For this review, take the finished solid that the model builds, in its own axes (mm). A direction names the side the tool comes from. Give positions to 0.01 mm unless a question says otherwise; leave off trailing zeros. Loops run counter-clockwise (first coordinate to the right, second up) from the corner with the lowest first, then second, coordinate; pieces in that order, holes last. Notation, with made-up numbers: (-16.75, 0) -> (28.25, 0) arc R21 ccw to (28.25, 12) -> close; hole circle Ø11 at (54.25, 30). An arc over 180 degrees is marked (long way). Answer as CSV lines item,"result". Start each with the question number.
Item 1: For L1, parallel to X at y = 35, z = 42.5; L2, parallel to Y at x = 90, z = 13; L3, parallel to Z at x = 5, y = 9, list the stretches that pass through material, from the lowest coordinate up. Write a range as from..to.
Item 2: Add section C-C on y = 32. State the section outline as (x, z) points.
Item 3: Clearance check with flat-ended pins moving along their axes: P1, Ø12, axis at x = 75, z = 18.5, coming from the +Y side; P2, Ø2, axis at y = 50.5, z = 39.5, coming from the +X side; P3, Ø3, axis at x = 16, z = 32.5, coming from the +Y side. State where each tip first meets the part, or that it passes through.
Item 4: Machinability: for faces 5 (the face through (94, 32, 41)), 6 (the face through (60, 55, 25)), 7 (the face through (35, 35, 38)), 8 (the face through (82, 3, 25)), which of the approach directions +Z, -Z, +X, -X, +Y, -Y give a long, thin tool a straight path to every point of the face, cutting with its end or side? Answer none if there is none.
Item 5: The part is to be moulded in two halves that separate along Y. For faces 1 (the face through (56.51, 4.19, 24.65)), 2 (the face through (86.4, 32.3, 20.2)), 3 (the face through (80, 41, 45)), 4 (the face through (80, 48, 25)), say which applies: +Y half, -Y half, draft (parallel to the pull), parting line (faces both ways), or undercut.
Item 6: Add section D-D on x = 90. State the section outline as (y, z) points, plus the area to 3 significant figures.
Item 7: Add section A-A on z = 34. State the section outline as (x, y) points, plus the area to 3 significant figures.
Item 8: Add section B-B on z = 8.5. State the section outline as (x, y) points.
```python
from build123d import *

# Parameters (mm, degrees)
BOSS_EXTRUDE1_DEPTH     = 50
SKETCH1_R               = 5
BOSS_EXTRUDE1_2_DEPTH   = 50
SKETCH1_5_R             = 4.5
BOSS_EXTRUDE2_DEPTH     = 41
BOSS_EXTRUDE3_DEPTH     = 30
BOSS_EXTRUDE4_DEPTH     = 38
CUT_EXTRUDE1_DEPTH      = 30
CUT_EXTRUDE2_DEPTH      = 101.344406919
CUT_EXTRUDE2_DEPTH_BACK = 101.344406919


with BuildPart() as part:
    # Sketch1 → Boss-Extrude1 (new body)
    with BuildSketch(Plane.XY):
        with BuildLine():
            Line((80, 48), (60, 48))
            Line((60, 48), (60, 63))
            Line((60, 63), (54.540446486, 63))
            Line((54.540446486, 63), (29.580398915, 63))
            Line((29.580398915, 63), (29.580398915, 60))
            ThreePointArc((29.580398915, 60), (54.037106954, 29.816426724), (19.438547859, 12.149554553))
            ThreePointArc((19.438547859, 12.149554553), (17.041767653, 13.371714676), (14.790199458, 14.844355629))
            ThreePointArc((14.790199458, 14.844355629), (7.781673687, 11.241937061), (0, 10))
            Line((0, 10), (0, 0))
            Line((0, 0), (45, 0))
            Line((45, 0), (68.339650933, 8.494938218))
            ThreePointArc((68.339650933, 8.494938218), (73.924248506, 8.860972081), (78.830920178, 6.169079822))
            Line((78.830920178, 6.169079822), (85, 0))
            Line((85, 0), (100, 0))
            Line((100, 0), (100, 15))
            ThreePointArc((100, 15), (85.857864376, 20.857864376), (80, 35))
            Line((80, 35), (80, 48))
        make_face()
    extrude(amount=BOSS_EXTRUDE1_DEPTH)

    # Sketch1_5 → Boss-Extrude2 (add)
    with BuildSketch(Plane.XY):
        with BuildLine():
            Line((100, 48), (80, 48))
            Line((80, 48), (80, 35))
            ThreePointArc((80, 35), (85.857864376, 20.857864376), (100, 15))
            Line((100, 15), (100, 48))
        make_face()
        with Locations((90, 35)):
            Circle(SKETCH1_5_R, mode=Mode.SUBTRACT)
    extrude(amount=BOSS_EXTRUDE2_DEPTH)

    # Sketch1_6 → Boss-Extrude3 (add)
    with BuildSketch(Plane.XY):
        with BuildLine():
            ThreePointArc((19.438547859, 12.149554553), (54.037106954, 29.816426724), (29.580398915, 60))
            Line((29.580398915, 60), (29.580398915, 45))
            ThreePointArc((29.580398915, 45), (39.560207875, 34.364851879), (28.312667533, 25.080682627))
            ThreePointArc((28.312667533, 25.080682627), (24.735564703, 18.024964247), (19.438547859, 12.149554553))
        make_face()
    extrude(amount=BOSS_EXTRUDE3_DEPTH)



with BuildPart() as body_2:
    # Sketch1 → Boss-Extrude1 2 (new body)
    with BuildSketch(Plane.XY):
        with Locations((29.580398915, 35)):
            Circle(SKETCH1_R)
    extrude(amount=BOSS_EXTRUDE1_2_DEPTH)


with BuildPart() as part_1:
    add(part.part)

    add(body_2.part)  # Boss-Extrude4 merges body 2
    # Sketch1_7 → Boss-Extrude4 (add)
    with BuildSketch(Plane.XY):
        with BuildLine():
            ThreePointArc((28.312667533, 25.080682627), (39.560207875, 34.364851879), (29.580398915, 45))
            Line((29.580398915, 45), (29.580398915, 40))
            ThreePointArc((29.580398915, 40), (33.115932821, 38.535533906), (34.580398915, 35))
            ThreePointArc((34.580398915, 35), (33.115932821, 31.464466094), (29.580398915, 30))
            ThreePointArc((29.580398915, 30), (29.050846917, 27.513459181), (28.312667533, 25.080682627))
        make_face()
    extrude(amount=BOSS_EXTRUDE4_DEPTH)

    # Sketch4 → Cut-Extrude1 (cut)
    with BuildSketch(Plane.XY):
        with BuildLine():
            Line((0, 10), (0, 35))
            Line((0, 35), (24.580398915, 35))
            ThreePointArc((24.580398915, 35), (26.04486501, 31.464466094), (29.580398915, 30))
            ThreePointArc((29.580398915, 30), (19.364916731, 12.087121525), (0, 5))
            Line((0, 5), (0, 10))
        make_face()
    extrude(amount=CUT_EXTRUDE1_DEPTH, mode=Mode.SUBTRACT)

    # Sketch5 → Cut-Extrude2 (cut, two sides: drawn at the far end of the back side and taken through both)
    with BuildSketch(Plane(origin=(60, 0, 0), x_dir=(0, 0, -1), z_dir=(1, 0, 0)).offset(-CUT_EXTRUDE2_DEPTH_BACK)):
        Polygon((0, 45), (-6.551464217, 63), (0, 63), align=None)
    extrude(amount=CUT_EXTRUDE2_DEPTH + CUT_EXTRUDE2_DEPTH_BACK, mode=Mode.SUBTRACT)


solid = part_1.part
```
Computed values:
1,L1,"24.58..34.58, 54.58..80"
1,L2,"0..30.5, 39.5..48"
1,L3,"30..50"
2,outline,"(25.58, 0) -> (86.65, 0) -> (86.65, 41) -> (80.23, 41) -> (80.23, 50) -> (54.4, 50) -> (54.4, 30) -> (39.12, 30) -> (39.12, 38) -> (33.58, 38) -> (33.58, 50) -> (25.58, 50) -> close; (93.35, 0) -> (100, 0) -> (100, 41) -> (93.35, 41) -> close"
3,P1,"y = 48"
3,P2,"x = 60"
3,P3,"y = 14.84"
4,face 5,"+Z, +X, +Y"
4,face 6,"+Z, -Z, +X, +Y"
4,face 7,"+Z"
4,face 8,"+Z, -Z, -Y"
5,face 1,"-Y half"
5,face 2,"undercut"
5,face 3,"draft"
5,face 4,"+Y half"
6,outline,"(0, 0) -> (30.5, 0) -> (30.5, 41) -> (17.68, 41) -> (17.68, 50) -> (0, 50) -> close; (39.5, 0) -> (45, 0) -> (48, 1.09) -> (48, 41) -> (39.5, 41) -> close"
6,area,"1,760 mm²"
7,outline,"(0, 0) -> (45, 0) -> (68.34, 8.49) arc R10 cw to (78.83, 6.17) -> (85, 0) -> (100, 0) -> (100, 48) -> (60, 48) -> (60, 63) -> (29.58, 63) -> (29.58, 60) arc R25 cw (long way) to (14.79, 14.84) arc R25 cw to (0, 10) -> close; (28.31, 25.08) arc R10 ccw (long way) to (29.58, 45) -> (29.58, 40) arc R5 ccw to (29.58, 30) arc R30 cw to start; hole circle Ø9 at (90, 35)"
7,area,"3,130 mm²"
8,outline,"(0, 0) -> (45, 0) -> (68.34, 8.49) arc R10 cw to (78.83, 6.17) -> (85, 0) -> (100, 0) -> (100, 48) -> (60, 48) -> (60, 63) -> (29.58, 63) -> (29.58, 40) arc R5 ccw to (29.58, 30) arc R30 cw to (0, 5) -> close; hole circle Ø9 at (90, 35)"
